from build123d import *

# Parameters (mm, degrees)
SKETCH1_R           = 8
BOSS_EXTRUDE1_DEPTH = 3.5
SKETCH2_R           = 2
BOSS_EXTRUDE2_DEPTH = 11
SKETCH4_R           = 1.2
CUT_EXTRUDE1_DEPTH  = 4.5
SKETCH5_R           = 2.1
CUT_EXTRUDE2_DEPTH  = 2
CHAMFER2_SIZE       = 0.2
FILLET3_R           = 0.5
FILLET4_R           = 0.5


with BuildPart() as part:
    # Sketch1 → Boss-Extrude1 (new body)
    with BuildSketch(Plane(origin=(0, 0, 0), x_dir=(1, 0, 0), z_dir=(0, 1, 0))):
        Circle(SKETCH1_R)
    extrude(amount=BOSS_EXTRUDE1_DEPTH)

    # Sketch2 → Boss-Extrude2 (add)
    with BuildSketch(Plane(origin=(0, 3.5, 0), x_dir=(1, 0, 0), z_dir=(0, 1, 0))):
        Circle(SKETCH2_R)
    extrude(amount=BOSS_EXTRUDE2_DEPTH)

    # Sketch4 → Cut-Extrude1 (cut, through all)
    with BuildSketch(Plane(origin=(0, 3.5, 0), x_dir=(1, 0, 0), z_dir=(0, 1, 0))):
        with Locations((0, 4.5)):
            Circle(SKETCH4_R)
        with Locations((4.5, 0)):
            Circle(SKETCH4_R)
        with Locations((0, -4.5)):
            Circle(SKETCH4_R)
        with Locations((-4.5, 0)):
            Circle(SKETCH4_R)
    extrude(amount=-CUT_EXTRUDE1_DEPTH, mode=Mode.SUBTRACT)

    # Sketch5 → Cut-Extrude2 (cut)
    with BuildSketch(Plane(origin=(0, 3.5, 0), x_dir=(1, 0, 0), z_dir=(0, 1, 0))):
        with Locations((0, 4.5)):
            Circle(SKETCH5_R)
        with Locations((4.5, 0)):
            Circle(SKETCH5_R)
        with Locations((0, -4.5)):
            Circle(SKETCH5_R)
        with Locations((-4.5, 0)):
            Circle(SKETCH5_R)
    extrude(amount=-CUT_EXTRUDE2_DEPTH, mode=Mode.SUBTRACT)

    # Chamfer2
    chamfer2_edges = [part.edges().sort_by_distance(p)[0] for p in [
        (-2.1, 3.5, -4.5),
        (2.4, 3.5, 0),
        (-2.1, 3.5, 4.5),
        (-6.6, 3.5, 0),
    ]]
    chamfer(chamfer2_edges, length=CHAMFER2_SIZE)

    # Fillet3
    fillet3_edges = [part.edges().sort_by_distance(p)[0] for p in [
        (-2, 14.5, 0),
    ]]
    fillet(fillet3_edges, radius=FILLET3_R)

    # Fillet4
    fillet4_edges = [part.edges().sort_by_distance(p)[0] for p in [
        (-8, 0, 0),
        (-8, 3.5, 0),
    ]]
    fillet(fillet4_edges, radius=FILLET4_R)


solid = part.part
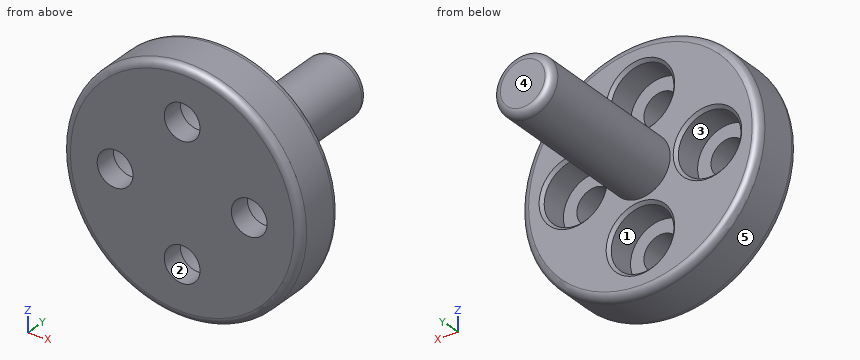
Work out the finished part from the listing and answer in its coordinate system (mm). Face numbers are marked on the shaded views. A direction names the side the tool comes from. Coordinates: 2 decimals unless noted, no trailing zeros. Order: outer loops, then holes, each group sorted by start corner. A loop starts at its lowest first (then second) coordinate and runs counter-clockwise, first axis right, second up. Notation, with made-up numbers: (-5, 16) - (13, 16) arc R20 cw to (13, 53) - close; hole circle Ø11 at (-25.5, -3.5). An arc over 180 degrees is marked (long way). Put each result on its own line as item: value. Start each with the question number.
1) For a pull along X with two mould halves and no side action, classify the marked faces 3, 4 and 5 as released by +X, released by -X, zero draft, split by the parting line, or undercut.
2) Find section C-C (y = 6.75). Give the vertices of the cut face in (x, z), plus the area to 3 significant figures.
3) Find the intervals of material crossed by line 1 (X direction, y = 2.95, z = 0); line 2 (X direction, y = 0.4, z = 4.5), in increasing order. Write a range as from..to.
4) For the marked faces 1 and 2, determine the directions among +Z, -Z, +X, -X, +Y, -Y from which every point of the face is accessible in a straight line to the end or side of a thin tool.
5) Flat-ended cylindrical pins translate along their axes: pin 1 (4 mm diameter, centred on x = 0, z = -4.5, fed in from -Y); pin 2 (3 mm diameter, centred on y = 2, z = -3.5, fed in from +X); pin 3 (4 mm diameter, centred on x = 0, z = -4.5, fed in from +Y); pin 4 (4 mm diameter, centred on x = 2.5, y = 2.5, fed in from +Z). Find the tip coordinate at first contact, or state that the pin passes through.
6) Find section A-A (z = 0). State how many separate pieces and enclosed holes the cut face has, plus the area to 3 significant figures.
Results list:
1. face 3: undercut
1. face 4: zero draft
1. face 5: split by the parting line
2. outline: circle Ø4 at (0, 0)
2. area: 12.6 mm^2
3. line 1: x = -8..-6.6, -2.4..2.4, 6.6..8
3. line 2: x = -6.6..-1.2, 1.2..6.6
4. face 1: +Y
4. face 2: +Y, -Y
5. pin 1: stops at y = 0
5. pin 2: stops at x = 7.75
5. pin 3: stops at y = 1.5
5. pin 4: stops at z = 7.98
6. separate pieces: 3
6. enclosed holes: 0
6. area: 75.6 mm^2
